Source: CAD feature listing. Evaluate the final solid. Frame: model axes, mm. A direction names the side the tool comes from. Round coordinates to 2 decimals unless told otherwise and drop trailing zeros. Write each loop counter-clockwise with the first axis right and the second up, starting at its lowest first coordinate (ties: lowest second). Pieces come first, ordered by that corner, then holes. Notation, with made-up numbers: (-13.75, 53) -> (-1.75, 53) arc R14 ccw to (-1.75, 59) -> close; hole circle Ø10 at (48, 72.25). An arc over 180 degrees is marked (long way). Put each result on its own line as item: value.
Autodesk Inventor part; units mm, degrees
ref_plane "YZ Plane" through (0, 0, 0) normal (1, 0, 0) x (0, 1, 0)
ref_plane "XZ Plane" through (0, 0, 0) normal (0, 1, 0) x (-1, 0, 0)
ref_plane "XY Plane" through (0, 0, 0) normal (0, 0, 1) x (1, 0, 0)
sketch "Sketch1" plane through (0, 0, 0) normal (0, 1, 0) x (-1, 0, 0)
  circle A0 centre (0, 0) radius 100.151
  line L0 (0, 0) -> (50.0755, -86.7333)
  line L1 (0, 0) -> (100.151, 0) construction
  line L2 (0, 0) -> (50.0755, 86.7333)
  line L3 (0, 0) -> (100.151, 0) construction
  line L4 (0, 0) -> (-100.151, 0)
  line L5 (50.0755, -86.7333) -> (100.0755, -86.7333) construction
  line L6 (50.0755, -86.7333) -> (24.5339, -97.0995)
  line L7 (50.0755, -86.7333) -> (100.0755, -86.7333) construction
  line L8 (71.8237, -69.7967) -> (50.0755, -86.7333)
  circle A1 centre (0, 0) radius 102.651
  line L9 (0, 0) -> (71.8237, -69.7967)
  line L10 (71.8237, -69.7967) -> (73.6166, -71.539)
  line L11 (0, 0) -> (24.5339, -97.0995)
  line L12 (24.5339, -97.0995) -> (25.1463, -99.5233)
  dimension "d0" = 200.302
  dimension "d1" = 60
  dimension "d2" = 60
  dimension "d8" = 205.302
extrude "Extrusion1" add sketch "Sketch1" along normal blind 40 contours L10 A1 L12 A0 picked at (67.2642, -76.2102)
sketch "Sketch2" plane through (0, 0, 0) normal (0, -1, 0) x (1, 0, 0)
  line L0 (-24.5339, -97.0995) -> (-25.1463, -99.5233)
  line L1 (-24.8401, -98.3114) -> (-21.9315, -99.0463)
  circle A0 centre (-21.9315, -99.0463) radius 1.5
  line L2 (-73.6166, -71.539) -> (-71.8237, -69.7967)
  line L3 (-72.7201, -70.6679) -> (-74.8716, -72.7586)
  line L4 (-74.8716, -72.7586) -> (-72.7201, -70.6679)
  line L5 (-72.7201, -70.6679) -> (-74.8109, -68.5164)
  circle A1 centre (-74.8109, -68.5164) radius 1.5
  circle A2 centre (-74.8109, -68.5164) radius 3
  arc A3 (-73.6166, -71.539) -> (-25.1463, -99.5233) centre (0, 0) ccw
  line L6 (-73.6166, -71.539) -> (-74.8109, -71.5164)
  arc A4 (-71.8237, -69.7967) -> (-24.5339, -97.0995) centre (0, 0) ccw
  line L7 (-71.8109, -68.5164) -> (-71.8237, -69.7967)
  circle A5 centre (-21.9315, -99.0463) radius 3
  line L8 (-21.9315, -99.0463) -> (-24.5296, -100.5463)
  line L9 (-21.9315, -99.0463) -> (-18.9315, -99.0463) construction
  line L10 (-24.5296, -100.5463) -> (-25.1463, -99.5233)
  arc A6 (-22.1585, -98.9889) -> (-21.9315, -99.0463) centre (-21.9315, -98.5684) ccw
  line L11 (-21.9315, -99.0463) -> (-22.9003, -97.4384)
  line L12 (-21.9315, -99.0463) -> (-20.0543, -99.0463) construction
  line L13 (-22.9003, -97.4384) -> (-23.4798, -96.4767)
  line L14 (-23.4798, -96.4767) -> (-24.5339, -97.0995)
  point P0 (0, 0)
  dimension "d12" = 3
  dimension "d13" = 3
  dimension "d14" = 3
  dimension "d15" = 210
  dimension "d16" = 121.07
extrude "Extrusion2" add sketch "Sketch2" against normal blind 3 contours L14 A5 L0 | L7 L2 A2 | A5 L10 L0 | A5 L13 L11 A0 L1 | L1 A0 L8 A5 | A5 L8 A0 L11 L13 | A0 L11 L1 | L1 A6 L8 A0 | L2 L6 A2 | A2 | L1 A6 | A0 L8 L11
sketch "Sketch3" plane through (0, 3, 0) normal (0, 1, 0) x (1, 0, 0)
  arc A0 (-23.4798, 96.4767) -> (-24.5296, 100.5463) centre (-21.9315, 99.0463) ccw
  circle A1 centre (-21.9315, 99.0463) radius 1.5
  point P0 (0, 0)
  dimension "d19" = 3
extrude "Extrusion3" cut sketch "Sketch3" against normal blind 3
sketch "Sketch4" plane through (-25.1463, 3, -99.5233) normal (0.9695, 0, -0.245) x (-0.245, 0, -0.9695)
  point P0 (-102.651, -3)
sketch "Sketch5" plane through (0, 40, 0) normal (0, 1, 0) x (1, 0, 0)
  circle A0 centre (-74.8109, 68.5164) radius 1.5
  circle A1 centre (-21.9315, 99.0463) radius 1.5
  line L0 (-74.8109, 68.5164) -> (-21.9315, 99.0463)
  circle A2 centre (-48.3712, 83.7814) radius 1.75
  circle A3 centre (-48.3712, 83.7814) radius 4
  line L1 (-44.9071, 85.7814) -> (-46.5714, 88.6641)
  arc A4 (-24.5339, 97.0995) -> (-71.8237, 69.7967) centre (0, 0) ccw
  line L2 (-51.8353, 81.7814) -> (-53.4996, 84.6641)
  line L3 (-46.5714, 88.6641) -> (-50.0755, 88.3957)
  line L4 (-50.0755, 88.3957) -> (-52.8557, 86.4967)
  line L5 (-52.8557, 86.4967) -> (-53.4996, 84.6641)
  point P0 (0, 0)
  dimension "d22" = 3.5
  dimension "d23" = 8
extrude "Extrusion4" add sketch "Sketch5" against normal blind 3 contours A3 A4 L0 A2 | L0 A2 A3 | L2 A4 A3 | L5 L4 L3 A4 A3 | A2 L0 | L0 A2 | A3 A4 | A3 A4 L1
sketch "Sketch6" plane through (0, 40, 0) normal (0, 1, 0) x (1, 0, 0)
  arc A0 (-51.8353, 81.7814) -> (-44.9071, 85.7814) centre (-48.3712, 83.7814) ccw
  circle A1 centre (-48.3712, 83.7814) radius 1.75
  point P0 (0, 0)
  dimension "d26" = 3.5
extrude "Extrusion5" cut sketch "Sketch6" against normal blind 3
sketch "Sketch7" plane through (0, 40, 0) normal (0, 1, 0) x (1, 0, 0)
  point P0 (0, 0)
sketch "Sketch8" plane through (0, 40, 0) normal (0, 1, 0) x (1, 0, 0)
  line L0 (0, 0) -> (-59.2945, 80.7117)
  arc A0 (-53.4996, 84.6641) -> (-71.8237, 69.7967) centre (0, 0) ccw
sketch "Sketch10" plane through (0, 40, 0) normal (0, 1, 0) x (1, 0, 0)
  circle A0 centre (-21.9315, 99.0463) radius 1.5
  circle A1 centre (-74.8109, 68.5164) radius 1.5
  line L0 (-21.9315, 99.0463) -> (-74.8109, 68.5164)
  line L1 (-48.3712, 83.7814) -> (0, 0)
  line L2 (-48.3712, 83.7814) -> (-44.0002, 76.2106)
  circle A2 centre (-44.0002, 76.2106) radius 1.75
  circle A3 centre (-44.0002, 76.2106) radius 4.01
  line L3 (-47.6057, 74.4556) -> (-52.7918, 83.4382)
  line L4 (-51.8353, 81.7814) -> (-53.4996, 84.6641)
  line L5 (-40.6779, 78.4561) -> (-45.4294, 86.686)
  line L6 (-45.4294, 86.686) -> (-49.4653, 86.686)
  line L7 (-49.4653, 86.686) -> (-52.7918, 83.4382)
  dimension "d30" = 96.7424
  dimension "d31" = 8.742
  dimension "d32" = 3.5
extrude "Extrusion6" add sketch "Sketch10" along normal blind 20 and the other way blind 3 contours L5 A3 L1 L0 | L0 L3 L7 L6 L5 | L1 A3 L3 L0 | A3 L1 A2 | L1 A2 A3
sketch "Sketch11" plane through (0, 40, 0) normal (0, 1, 0) x (1, 0, 0)
  arc A0 (-24.5339, 97.0995) -> (-46.5714, 88.6641) centre (0, 0) ccw
  arc A1 (-24.5339, 97.0995) -> (-46.5714, 88.6641) centre (0, 0) ccw
  line L0 (-53.4996, 84.6641) -> (-52.7918, 83.4382)
  line L1 (-73.6166, 71.539) -> (-71.8237, 69.7967)
  arc A2 (-53.4996, 84.6641) -> (-71.8237, 69.7967) centre (0, 0) ccw
  arc A3 (-25.1463, 99.5233) -> (-73.6166, 71.539) centre (0, 0) ccw
  arc A4 (-25.1463, 99.5233) -> (-73.6166, 71.539) centre (0, 0) ccw
  line L2 (-25.1463, 99.5233) -> (-24.5339, 97.0995)
  line L3 (-73.6166, 71.539) -> (-71.8237, 69.7967)
  line L4 (-53.4996, 84.6641) -> (-52.7918, 83.4382)
  line L5 (-52.7918, 83.4382) -> (-49.4653, 86.686)
  line L6 (-52.7918, 83.4382) -> (-49.4653, 86.686)
  line L7 (-49.4653, 86.686) -> (-45.4294, 86.686)
  line L8 (-49.4653, 86.686) -> (-45.4294, 86.686)
  line L9 (-45.4294, 86.686) -> (-46.5714, 88.6641)
  point P0 (0, 0)
  dimension "d37" = 100.151
extrude "Extrusion7" add sketch "Sketch11" along normal blind 20
sketch "Sketch12" plane through (0, 37, 0) normal (0, -1, 0) x (1, 0, 0)
  line L0 (-47.6057, -74.4556) -> (-53.4996, -84.6641)
  line L1 (-45.4294, -86.686) -> (-46.5714, -88.6641)
  arc A0 (-53.4996, -84.6641) -> (-46.5714, -88.6641) centre (0, 0) ccw
  line L2 (-53.4996, -84.6641) -> (-54.9814, -68.7673)
  line L3 (-54.9814, -68.7673) -> (-38.2505, -67.5322)
  line L4 (-38.2505, -67.5322) -> (-32.7507, -81.5808)
  line L5 (-32.7507, -81.5808) -> (-46.5714, -88.6641)
  point P0 (0, 0)
extrude "Extrusion8" cut sketch "Sketch12" against normal blind 20
properties part number "Wheel Guard1"
Q1. Pin query (flat end, axial travel): pin 1 (12 mm diameter, centred on x = -69, z = -72.5, fed in from -Y); pin 2 (1.5 mm diameter, centred on y = 34, z = -69.5, fed in from -X); pin 3 (3 mm diameter, centred on y = 52, z = -69.5, fed in from +X); pin 4 (5 mm diameter, centred on y = 7, z = -98, fed in from +X). Return the tip coordinate at first contact, or that it passes through.
Ans:
pin 1: stops at y = 0
pin 2: stops at x = -72.29
pin 3: stops at x = -70.63
pin 4: stops at x = -24.53
Q2. Material intervals for line 1 (Y direction, x = -49, z = -85); line 2 (X direction, y = 55.5, z = -71); line 3 (X direction, y = 52, z = -93), sorted ascending. Write a range as [from, to].
Ans:
line 1: y = [57, 60]
line 2: x = [-73.06, -70.63]
line 3: x = [-43.45, -37.16]
Q3. Draft query along X for faces 5 (the flat face through (-72.71, 31.1, -70.66)), 6 (the flat face through (-47, 60, -84)), 7 (the cylindrical face through (-76.31, 1.48, -68.45)). Return one class per face: +X half, -X half, draft (parallel to the pull), parting line (faces both ways), or undercut.
Ans:
face 5: -X half
face 6: draft
face 7: undercut
Q4. Cut plane A-A on z = -79.5. Output: boundary loops of the cut face in (x, y), and give its area (3 significant figures).
Ans:
outline: (-64.94, 0) -> (-60.91, 0) -> (-60.91, 60) -> (-64.94, 60) -> close; (-50.52, 57) -> (-41.28, 57) -> (-41.28, 60) -> (-50.52, 60) -> close
area: 269 mm^2
Q5. Cut plane B-B on y = 44. Output: boundary loops of the cut face in (x, z).
Ans:
outline: (-73.62, -71.54) arc R102.65 ccw to (-25.15, -99.52) -> (-24.53, -97.1) arc R100.15 cw to (-46.57, -88.66) arc R100.15 cw to (-53.5, -84.66) arc R100.15 cw to (-71.82, -69.8) -> close
Q6. Cut plane C-C on x = -41.5. Output: boundary loops of the cut face in (y, z).
Ans:
outline: (0, -93.89) -> (60, -93.89) -> (60, -91.15) -> (0, -91.15) -> close; (57, -79.88) -> (60, -79.88) -> (60, -73.08) -> (57, -73.08) -> close
Q7. Cut plane D-D on z = -87.5. Output: boundary loops of the cut face in (x, y), and give its area (3 significant figures).
Ans:
outline: (-53.67, 0) -> (-48.72, 0) -> (-48.72, 57) -> (-45.9, 57) -> (-45.9, 60) -> (-53.67, 60) -> close
area: 306 mm^2
Q8. Reachability of faces 1 (the flat face through (-24.844, 31.101, -98.328)), 2 (the flat face through (-74, 3, -67)), 3 (the flat face through (-53, 0, -86)), 4 (the flat face through (-47, 57, -80)) from +Z, -Z, +X, -X, +Y, -Y: full face, straight path, thin tool, end or side. Return the list, or none.
Ans:
face 1: -Z, +X, +Y
face 2: +Z, -X, +Y
face 3: +Z, -Z, +X, -X, -Y
face 4: +Z, +X, -Y
